Autodesk Inventor part; units mm, degrees
ref_plane "YZ Plane" through (0, 0, 0) normal (1, 0, 0) x (0, 1, 0)
ref_plane "XZ Plane" through (0, 0, 0) normal (0, 1, 0) x (-1, 0, 0)
ref_plane "XY Plane" through (0, 0, 0) normal (0, 0, 1) x (1, 0, 0)
sketch "Sketch1" plane through (0, 0, 0) normal (0, 0, 1) x (1, 0, 0)
  line L0 (0, 0) -> (0, -0.45)
  line L1 (0, -0.45) -> (-0.35, -0.45)
  line L2 (0, 0) -> (-0.35, 0)
  arc A0 (-0.35, -0.45) -> (-0.5, -0.6) centre (-0.35, -0.6) ccw
  arc A1 (-0.35, 0) -> (-0.95, -0.6) centre (-0.35, -0.6) ccw
  line L3 (-0.95, -0.6) -> (-0.95, -7.9)
  line L4 (-0.95, -7.9) -> (-0.5, -7.9)
  line L5 (-0.5, -7.9) -> (-0.5, -0.6)
  dimension "d0" = 0.45
  dimension "d2" = 7.9
  dimension "d3" = 0.95
  dimension "d4" = 0.6
extrude "Extrusion1" add sketch "Sketch1" along normal blind 2.5
fillet "Fillet1" radius 1.25 2 edges at (-0.725, -7.9, 2.5) (-0.725, -7.9, 0)
properties material "Brass, Soft Yellow"
Input: part model. Units: mm. Frame: model coordinates. A direction names the side the tool comes from. Coordinates: 2 decimals unless noted, no trailing zeros. Loops run counter-clockwise (first coordinate to the right, second up) from the corner with the lowest first, then second, coordinate; pieces in that order, holes last. Notation, with made-up numbers: M -6.75,21 L 22.25,21 A29 cw 22.25,49 Z; hole C -13,85 d8. An arc over 180 degrees is marked long. Answer in a Markdown table with one row per item.
1. Material intervals for line 1 (Y direction, x = -0.2, z = 2.2); line 2 (X direction, y = -6, z = 1.15); line 3 (Y direction, x = -0.7, z = 2.35), sorted ascending.
Response:
| item | result |
|---|---|
| line 1 | y = -0.45 to 0 |
| line 2 | x = -0.95 to -0.5 |
| line 3 | y = -7.24 to -0.11 |
2. Section A-A, the plane z = 1.75. Output: boundary loops of the cut face in (x, y).
Response:
| item | result |
|---|---|
| outline | M -0.95,-7.8 L -0.5,-7.8 L -0.5,-0.6 A0.15 cw -0.35,-0.45 L 0,-0.45 L 0,0 L -0.35,0 A0.6 ccw -0.95,-0.6 Z |
3. Section C-C, the plane y = -2. Output: boundary loops of the cut face in (x, z).
Response:
| item | result |
|---|---|
| outline | M -0.95,0 L -0.5,0 L -0.5,2.5 L -0.95,2.5 Z |
4. Section D-D, the plane z = 0.4. Output: boundary loops of the cut face in (x, y), then the cut area to 3 significant figures.
Response:
| item | result |
|---|---|
| outline | M -0.95,-7.57 L -0.5,-7.57 L -0.5,-0.6 A0.15 cw -0.35,-0.45 L 0,-0.45 L 0,0 L -0.35,0 A0.6 ccw -0.95,-0.6 Z |
| area | 3.56 mm2 |
5. Reachability of faces 1 (the flat face through (-0.95, -4, 1)), 2 (the flat face through (-0.5, -4, 1)) from +Z, -Z, +X, -X, +Y, -Y: full face, straight path, thin tool, end or side. Return the list, or none.
Response:
| item | result |
|---|---|
| face 1 | +Z, -Z, -X, +Y, -Y |
| face 2 | +Z, -Z, +X, -Y |
6. First-contact query: pin 1 (0.8 mm diameter, centred on y = -5, z = 1, fed in from +X). Flat tip, straight axial feed; report the tip coordinate or a pass-through.
Response:
| item | result |
|---|---|
| pin 1 | stops at x = -0.5 |
